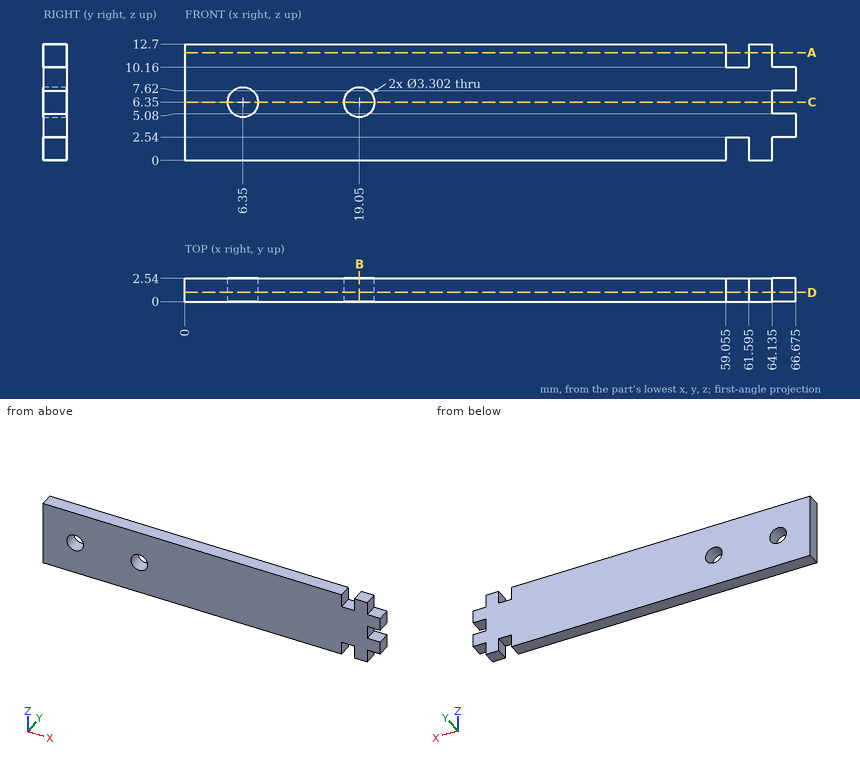
Job drawing, mm, ordinate dimensions from the low corner. One solid piece. Round coordinates to 2 decimals unless told otherwise and drop trailing zeros. Loops run counter-clockwise (first coordinate to the right, second up) from the corner with the lowest first, then second, coordinate; pieces in that order, holes last.
(1) Cut at A-A (z = 11.75). Give the cut face in (x, y) (3 decimals).
(2) Cut at C-C (z = 6.35). Give the cut face in (x, y) (3 decimals), plus the area to 3 significant figures.
(3) Cut at B-B (x = 19.05). Give the cut face in (y, z).
(4) Cut at D-D (y = 1). Give the cut face in (x, z) (3 decimals).
(5) Drop flat-ended pins along their axis: pin 1 (0.8 mm diameter, centred on x = 60, y = 2, fed in from -Z); pin 2 (1.3 mm diameter, centred on y = 1, z = 1.5, fed in from +X) (3 decimals); pin 3 (1.3 mm diameter, centred on x = 65, y = 1, fed in from +Z). Give the stop position or say it passes through.
(6) Wall check: line 1 along X through (y, z) = (1.2, 6.35) (3 decimals); line 2 along X through (y, z) = (0.85, 11.5) (3 decimals); line 3 along X through (y, z) = (1.4, 7.5) (3 decimals). Give the ranges that are in metal, low to high.
Findings below:
1. outline: (0, 0) - (59.055, 0) - (59.055, 2.54) - (0, 2.54) - close; (61.595, 0) - (64.135, 0) - (64.135, 2.54) - (61.595, 2.54) - close
2. outline: (0, 0) - (4.699, 0) - (4.699, 2.54) - (0, 2.54) - close; (8.001, 0) - (17.399, 0) - (17.399, 2.54) - (8.001, 2.54) - close; (20.701, 0) - (64.135, 0) - (64.135, 2.54) - (20.701, 2.54) - close
2. area: 146 mm2
3. outline: (0, 0) - (2.54, 0) - (2.54, 4.7) - (0, 4.7) - close; (0, 8) - (2.54, 8) - (2.54, 12.7) - (0, 12.7) - close
4. outline: (0, 0) - (59.055, 0) - (59.055, 2.54) - (61.595, 2.54) - (61.595, 0) - (64.135, 0) - (64.135, 2.54) - (66.675, 2.54) - (66.675, 5.08) - (64.135, 5.08) - (64.135, 7.62) - (66.675, 7.62) - (66.675, 10.16) - (64.135, 10.16) - (64.135, 12.7) - (61.595, 12.7) - (61.595, 10.16) - (59.055, 10.16) - (59.055, 12.7) - (0, 12.7) - close; hole circle Ø3.302 at (6.35, 6.35); hole circle Ø3.302 at (19.05, 6.35)
5. pin 1: stops at z = 2.54
5. pin 2: stops at x = 64.135
5. pin 3: stops at z = 10.16
6. line 1: x = 0 to 4.699, 8.001 to 17.399, 20.701 to 64.135
6. line 2: x = 0 to 59.055, 61.595 to 64.135
6. line 3: x = 0 to 5.165, 7.535 to 17.865, 20.235 to 64.135
